The listing builds one solid part. Answer for the finished solid, in the listing's coordinates (mm). Face numbers are marked on the shaded views. A direction names the side the tool comes from. Coordinates: 2 decimals unless noted, no trailing zeros. Write each loop counter-clockwise with the first axis right and the second up, starting at its lowest first coordinate (ties: lowest second). Pieces come first, ordered by that corner, then holes.
(1) For a pull along Z with two mould halves and no side action, classify the marked faces 3 and 4 as +Z half, -Z half, draft (parallel to the pull), parting line (faces both ways), or undercut.
(2) The part is cut by section A-A on x = 73.15. Determine the outline of the cut face in (y, z), plus the area to 3 significant figures.
(3) Straight lines are drawn through the part: line 1 (X direction, y = 7.5, z = -56); line 2 (Z direction, x = 73.5, y = 0.75); line 3 (X direction, y = 3.25, z = -74). For each, find the intervals that lie inside material, in ascending order.
(4) Which of the six approach directions +Z, -Z, +X, -X, +Y, -Y give full straight-line access (tool end or side, diameter ignored) to the marked faces 1 and 2?
(5) Given P1, Ø2, axis at x = 60.5, z = -40, coming from the +Y side; P2, Ø2.5, axis at y = 5, z = -48.5, coming from the -X side; P3, Ø0.7, axis at x = 3, y = 8, coming from the -Z side, each flat-ended and moving along its own axis, determine where each tip first touches the part or whether it passes through.
(6) The part is cut by section D-D on z = -41. Determine the outline of the cut face in (x, y), plus the area to 3 significant figures.
(7) The part is cut by section B-B on z = -83. Determine the outline of the cut face in (x, y), plus the area to 3 significant figures.
(8) The part is cut by section C-C on y = 8. Give the number of separate pieces and of enclosed holes in the cut face, plus the area to 3 significant figures.
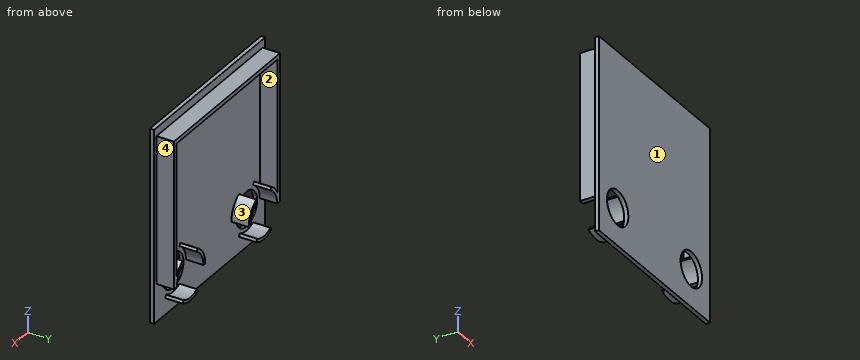
Autodesk Inventor part; units mm, degrees
ref_plane "YZ Plane" through (0, 0, 0) normal (1, 0, 0) x (0, 1, 0)
ref_plane "XZ Plane" through (0, 0, 0) normal (0, 1, 0) x (-1, 0, 0)
ref_plane "XY Plane" through (0, 0, 0) normal (0, 0, 1) x (1, 0, 0)
sketch "Sketch1" plane through (0, 0, 0) normal (0, 1, 0) x (-1, 0, 0)
  line L0 (0, 0) -> (-88, 0)
  line L1 (-88, 0) -> (-88, -94)
  line L2 (-88, -94) -> (0, -94)
  line L3 (0, -94) -> (0, 0)
  line L4 (0, -94) -> (0, -75.65)
  line L5 (0, -94) -> (-14.85, -94)
  circle A0 centre (-14.85, -75.65) radius 8.45
  line L6 (-44, -88.9444) -> (-44, -54.2543) construction
  circle A1 centre (-73.15, -75.65) radius 8.45
  dimension "d0" = 88
  dimension "d1" = 94
  dimension "d2" = 18.35
  dimension "d3" = 14.85
  dimension "d4" = 16.9
  dimension "d48" = 16.9
extrude "Extrusion1" add sketch "Sketch1" along normal blind 2
sketch "Sketch3" plane through (0, 2, 0) normal (0, 1, 0) x (1, 0, 0)
  circle A0 centre (73.15, 75.65) radius 8.45 construction
  circle A1 centre (14.85, 75.65) radius 8.45 construction
  line L0 (0, 0) -> (4, 0) construction
  line L1 (4, 0) -> (4, 6) construction
  line L2 (4, 6) -> (0, 6) construction
  line L3 (0, 6) -> (0, 0) construction
  line L4 (88, 0) -> (84, 0) construction
  line L5 (84, 0) -> (84, 6) construction
  line L6 (84, 6) -> (88, 6) construction
  line L7 (88, 6) -> (88, 0) construction
  line L8 (4, 6) -> (2, 6) construction
  line L9 (2, 6) -> (2, 4) construction
  line L10 (2, 4) -> (4, 4) construction
  line L11 (4, 4) -> (4, 6) construction
  line L12 (2, 4) -> (6, 4)
  line L13 (6, 4) -> (6, 6)
  line L14 (6, 6) -> (2, 6)
  line L15 (2, 6) -> (2, 4)
  line L16 (2, 4) -> (4, 4)
  line L17 (4, 4) -> (4, 8)
  line L18 (4, 8) -> (2, 8)
  line L19 (2, 8) -> (2, 4)
  line L20 (86, 4) -> (82, 4)
  line L21 (82, 4) -> (82, 4)
  line L22 (82, 4) -> (86, 4)
  line L23 (86, 4) -> (86, 4)
  line L24 (86, 4) -> (84, 4)
  line L25 (84, 4) -> (84, 8)
  line L26 (84, 8) -> (86, 8)
  line L27 (86, 8) -> (86, 4)
  line L28 (44, 4.3599) -> (37, 4.3599) construction
  line L29 (88, -1) -> (0, -1) construction
  line L30 (37, -1) -> (51, -1) construction
  line L31 (51, -1) -> (51, 0) construction
  line L32 (51, 0) -> (37, 0) construction
  line L33 (37, 0) -> (37, -1) construction
  line L34 (37, -1) -> (51, -1)
  line L35 (51, -1) -> (51, 0)
  line L36 (51, 0) -> (37, 0)
  line L37 (37, 0) -> (37, -1)
  line L38 (0, 95) -> (88, 95)
  line L39 (37, 95) -> (51, 95)
  line L40 (51, 95) -> (51, 94)
  line L41 (51, 94) -> (37, 94)
  line L42 (37, 94) -> (37, 95)
  circle A2 centre (14.85, 75.65) radius 10.45
  circle A3 centre (14.85, 75.65) radius 11.95
  line L43 (14.85, 75.65) -> (26.8, 75.65) construction
  line L44 (14.85, 75.65) -> (20.825, 85.999) construction
  line L45 (14.85, 75.65) -> (8.875, 85.999) construction
  line L46 (14.85, 75.65) -> (2.9, 75.65) construction
  line L47 (14.85, 75.65) -> (8.875, 65.301) construction
  line L48 (14.85, 75.65) -> (20.825, 65.301) construction
  line L49 (9.625, 84.7) -> (8.875, 85.999) construction
  line L50 (9.625, 84.7) -> (8.875, 85.999)
  line L51 (20.825, 85.999) -> (20.075, 84.7)
  line L52 (25.3, 75.65) -> (26.8, 75.65)
  line L53 (20.825, 65.301) -> (20.075, 66.6)
  line L54 (9.625, 66.6) -> (8.875, 65.301)
  line L55 (4.4, 75.65) -> (2.9, 75.65)
  line L56 (44, 84.7433) -> (44, 74.6259) construction
  circle A4 centre (73.15, 75.65) radius 8.45 construction
  circle A5 centre (73.15, 75.65) radius 10.45
  circle A6 centre (73.15, 75.65) radius 11.95
  line L57 (73.15, 75.65) -> (61.2, 75.65) construction
  line L58 (73.15, 75.65) -> (67.175, 85.999) construction
  line L59 (73.15, 75.65) -> (79.125, 85.999) construction
  line L60 (73.15, 75.65) -> (85.1, 75.65) construction
  line L61 (73.15, 75.65) -> (79.125, 65.301) construction
  line L62 (73.15, 75.65) -> (67.175, 65.301) construction
  line L63 (78.375, 84.7) -> (79.125, 85.999) construction
  line L64 (78.375, 84.7) -> (79.125, 85.999)
  line L65 (67.175, 85.999) -> (67.925, 84.7)
  line L66 (62.7, 75.65) -> (61.2, 75.65)
  line L67 (67.175, 65.301) -> (67.925, 66.6)
  line L68 (78.375, 66.6) -> (79.125, 65.301)
  line L69 (83.6, 75.65) -> (85.1, 75.65)
  line L70 (86, 4) -> (82, 4)
  line L71 (82, 4) -> (82, 6)
  line L72 (82, 6) -> (86, 6)
  line L73 (86, 6) -> (86, 4)
  point P0 (2, 4)
  point P1 (4, 6)
  point P2 (84, 4)
  point P3 (67.175, 65.301)
  point P4 (79.125, 65.301)
  point P5 (2.9, 75.65)
  point P6 (8.875, 65.301)
  point P7 (20.825, 65.301)
  point P8 (84, 6)
  dimension "d11" = 4
  dimension "d12" = 6
  dimension "d13" = 4
  dimension "d14" = 6
  dimension "d15" = 2
  dimension "d16" = 2
  dimension "d17" = 4
  dimension "d18" = 4
  dimension "d19" = 4
  dimension "d20" = 2
  dimension "d21" = 4
  dimension "d22" = 7
  dimension "d23" = 14
  dimension "d24" = 14
  dimension "d25" = 1
  dimension "d26" = 2
  dimension "d27" = 1.5
  dimension "d30" = 360
extrude "Extrusion3" add sketch "Sketch3" along normal blind 8.5 contours L15 L14 L17 L12 | L17 L14 L13 L12 | L19 L18 L17 L14 | L20 L25 L72 L27 | L20 L71 L72 L25 | L72 L25 L26 L27 | L52 A3 L53 A2 | A2 L50 A3 L51 | L54 A3 L55 A2 | L69 A6 L68 A5 | A5 L65 A6 L64 | L67 A6 L66 A5
sketch "Sketch6" plane through (0, 2, 0) normal (0, 1, 0) x (1, 0, 0)
  arc A0 (78.375, 84.7) -> (67.925, 84.7) centre (73.15, 75.65) ccw construction
  line L0 (67.925, 84.7) -> (67.175, 85.999) construction
  arc A1 (79.125, 85.999) -> (67.175, 85.999) centre (73.15, 75.65) ccw construction
  line L1 (79.125, 85.999) -> (78.375, 84.7) construction
  line L2 (2, 8) -> (4, 8) construction
  line L3 (4, 8) -> (4, 6) construction
  line L4 (4, 6) -> (6, 6) construction
  line L5 (6, 6) -> (6, 4) construction
  line L6 (6, 4) -> (2, 4) construction
  line L7 (2, 4) -> (2, 8) construction
  line L8 (83.6, 75.65) -> (85.1, 75.65) construction
  arc A2 (79.125, 65.301) -> (85.1, 75.65) centre (73.15, 75.65) ccw construction
  line L9 (79.125, 65.301) -> (78.375, 66.6) construction
  arc A3 (78.375, 66.6) -> (83.6, 75.65) centre (73.15, 75.65) ccw construction
  line L10 (20.825, 85.999) -> (20.075, 84.7) construction
  arc A4 (20.075, 84.7) -> (9.625, 84.7) centre (14.85, 75.65) ccw construction
  line L11 (9.625, 84.7) -> (8.875, 85.999) construction
  arc A5 (20.825, 85.999) -> (8.875, 85.999) centre (14.85, 75.65) ccw construction
  line L12 (2.9, 75.65) -> (4.4, 75.65) construction
  arc A6 (4.4, 75.65) -> (9.625, 66.6) centre (14.85, 75.65) ccw construction
  line L13 (9.625, 66.6) -> (8.875, 65.301) construction
  arc A7 (2.9, 75.65) -> (8.875, 65.301) centre (14.85, 75.65) ccw construction
  line L14 (86, 8) -> (86, 4) construction
  line L15 (86, 4) -> (82, 4) construction
  line L16 (82, 4) -> (82, 6) construction
  line L17 (82, 6) -> (84, 6) construction
  line L18 (84, 6) -> (84, 8) construction
  line L19 (84, 8) -> (86, 8) construction
  arc A8 (62.7, 75.65) -> (67.925, 66.6) centre (73.15, 75.65) ccw construction
  line L20 (67.925, 66.6) -> (67.175, 65.301) construction
  arc A9 (61.2, 75.65) -> (67.175, 65.301) centre (73.15, 75.65) ccw construction
  line L21 (61.2, 75.65) -> (62.7, 75.65) construction
  line L22 (25.3, 75.65) -> (26.8, 75.65) construction
  arc A10 (20.825, 65.301) -> (26.8, 75.65) centre (14.85, 75.65) ccw construction
  line L23 (20.825, 65.301) -> (20.075, 66.6) construction
  arc A11 (20.075, 66.6) -> (25.3, 75.65) centre (14.85, 75.65) ccw construction
  line L24 (88, 94) -> (0, 94) construction
  line L25 (0, 94) -> (0, 0) construction
  line L26 (0, 0) -> (88, 0) construction
  line L27 (88, 0) -> (88, 94) construction
  circle A12 centre (73.15, 75.65) radius 8.45 construction
  circle A13 centre (14.85, 75.65) radius 8.45 construction
  line L28 (6, 4) -> (82, 4) construction
  line L29 (82, 4) -> (82, 6) construction
  line L30 (82, 6) -> (6, 6) construction
  line L31 (6, 6) -> (6, 4) construction
  line L32 (86, 8) -> (84, 8) construction
  line L33 (84, 8) -> (84, 75.65) construction
  line L34 (84, 75.65) -> (86, 75.65) construction
  line L35 (86, 75.65) -> (86, 8) construction
  line L36 (2, 8) -> (4, 8) construction
  line L37 (4, 8) -> (4, 75.65) construction
  line L38 (4, 75.65) -> (2, 75.65) construction
  line L39 (2, 75.65) -> (2, 8) construction
  line L40 (2, 75.65) -> (4, 75.65)
  line L41 (4, 75.65) -> (4, 8)
  line L42 (4, 8) -> (2, 8)
  line L43 (2, 8) -> (2, 75.65)
  line L44 (6, 6) -> (82, 6)
  line L45 (82, 6) -> (82, 4)
  line L46 (82, 4) -> (6, 4)
  line L47 (6, 4) -> (6, 6)
  line L48 (84, 8) -> (86, 8)
  line L49 (86, 8) -> (86, 75.65)
  line L50 (86, 75.65) -> (84, 75.65)
  line L51 (84, 75.65) -> (84, 8)
  dimension "d44" = 2
  dimension "d45" = 2
extrude "Extrusion6" add sketch "Sketch6" along normal blind 8.5
properties part number "case_v1.1"
Model answer:
1. face 3: undercut
1. face 4: draft
2. outline: (0, -94) - (2, -94) - (2, -87.6) - (10.5, -87.6) - (10.5, -86.1) - (2, -86.1) - (2, -84.1) - (0, -84.1) - close; (0, -67.2) - (2, -67.2) - (2, -6) - (10.5, -6) - (10.5, -4) - (2, -4) - (2, 0) - (0, 0) - close
2. area: 184 mm2
3. line 1: x = 2 to 4, 84 to 86
3. line 2: z = -94 to -84.09, -67.21 to 0
3. line 3: x = 2 to 4.53, 25.17 to 26.69, 61.31 to 62.83, 83.47 to 86
4. face 1: +Z, -Z, +X, -X, -Y
4. face 2: +Y
5. P1: stops at y = 2
5. P2: stops at x = 2
5. P3: stops at z = -75.65
6. outline: (0, 0) - (88, 0) - (88, 2) - (86, 2) - (86, 10.5) - (84, 10.5) - (84, 2) - (4, 2) - (4, 10.5) - (2, 10.5) - (2, 2) - (0, 2) - close
6. area: 210 mm2
7. outline: (0, 0) - (10.68, 0) - (10.68, 2) - (0, 2) - close; (19.02, 0) - (68.98, 0) - (68.98, 2) - (19.02, 2) - close; (77.32, 0) - (88, 0) - (88, 2) - (77.32, 2) - close
7. area: 143 mm2
8. separate pieces: 5
8. enclosed holes: 0
8. area: 545 mm2
